```python
from build123d import *

# Parameters (mm, degrees)
BASE_FLANGE1_DEPTH = 2.5


# Sheet-metal steps are written as plain solids
with BuildPart() as part:
    # Sketch1 → Base-Flange1 (new body)
    with BuildSketch(Plane.XY):
        with BuildLine():
            Line((-134.197014838, 0), (131.813755418, 0))
            ThreePointArc((131.813755418, 0), (144.49230327, 2.810766389), (154.795088711, 10.716371709))
            Line((154.795088711, 10.716371709), (488.882789575, 408.866589455))
            ThreePointArc((488.882789575, 408.866589455), (495.894882012, 428.778240774), (488.055453139, 448.3789207))
            Line((488.055453139, 448.3789207), (411.771088084, 531.923752399))
            ThreePointArc((411.771088084, 531.923752399), (401.723678511, 539.143738745), (389.617091226, 541.695049445))
            Line((389.617091226, 541.695049445), (204.630312304, 541.695049445))
            ThreePointArc((204.630312304, 541.695049445), (191.371044435, 538.605861688), (180.842467764, 529.974503817))
            Line((180.842467764, 529.974503817), (-127.984859378, 128.084146569))
            ThreePointArc((-127.984859378, 128.084146569), (-132.601550886, 119.457791797), (-134.197014838, 109.804692197))
            Line((-134.197014838, 109.804692197), (-134.197014838, 92.304692197))
            ThreePointArc((-134.197014838, 92.304692197), (-121.697014838, 79.804692197), (-134.197014838, 67.304692197))
            Line((-134.197014838, 67.304692197), (-134.197014838, 0))
        make_face()
    extrude(amount=-BASE_FLANGE1_DEPTH)


solid = part.part
```
The model under review builds one solid part; all positions refer to its coordinate system, in mm. Round coordinates to 2 decimals unless told otherwise and drop trailing zeros. Order: outer loops, then holes, each group sorted by start corner. A loop starts at its lowest first (then second) coordinate and runs counter-clockwise, first axis right, second up.
Item 1: Add section C-C, the plane y = 338. State the section outline as (x, z) points.
Working result:
outline: (33.32, -2.5) - (429.42, -2.5) - (429.42, 0) - (33.32, 0) - close
Item 2: Add section B-B, the plane x = 21. State the section outline as (y, z) points.
Working result:
outline: (0, -2.5) - (321.96, -2.5) - (321.96, 0) - (0, 0) - close
Item 3: Add section A-A, the plane z = -0.4. State the section outline as (x, y) points, and give its area (3 significant figures).
Working result:
outline: (-134.2, 0) - (131.81, 0) arc R30 ccw to (154.8, 10.72) - (488.88, 408.87) arc R30 ccw to (488.06, 448.38) - (411.77, 531.92) arc R30 ccw to (389.62, 541.7) - (204.63, 541.7) arc R30 ccw to (180.84, 529.97) - (-127.98, 128.08) arc R30 ccw to (-134.2, 109.8) - (-134.2, 92.3) arc R12.5 cw to (-134.2, 67.3) - close
area: 195,000 mm2
Item 4: To check wall thickness, follow probe 1 along X at (y, z) = (396.5, -0.95); probe 2 along Y at (x, z) = (297, -2); probe 3 along Y at (x, z) = (92, -0.85). State the ranges of each line that lie inside material, in increasing order.
Working result:
probe 1: x = 78.28 to 478.51
probe 2: y = 180.19 to 541.7
probe 3: y = 0 to 414.36
Item 5: For pin 1 (1 mm diameter, centred on y = 448.5, z = -2, fed in from +X); pin 2 (1.5 mm diameter, centred on y = 109.5, z = -1, fed in from +X), all flat-tipped, find the tip position at first contact; note any pin that passes through.
Working result:
pin 1: stops at x = 488.4
pin 2: stops at x = 238.31
